Build history of the part. All positions in model axes, mm. A direction names the side the tool comes from. Give positions to 0.01 mm unless a question says otherwise; leave off trailing zeros. Write each loop counter-clockwise with the first axis right and the second up, starting at its lowest first coordinate (ties: lowest second). Pieces come first, ordered by that corner, then holes. Notation, with made-up numbers: M 83,24 L 93,24 A25 cw 93,60 Z; hole C 40.25,64.25 d2. An arc over 180 degrees is marked long. One line per item, written item: value. Start each with the question number.
from build123d import *

# Parameters (mm, degrees)
PAD_DEPTH       = 36.55
SKETCH001_R     = 24.260062
PAD001_DEPTH    = 2
PAD002_DEPTH    = 8
PAD003_START    = 34.55
SKETCH005_R     = 22
SKETCH005_R_2   = 19
PAD003_DEPTH    = 2
SKETCH002_W     = 60
SKETCH002_H     = 10
POCKET002_DEPTH = 36.551
POCKET003_START = 8
SKETCH003_W     = 14
SKETCH003_H     = 60
POCKET003_DEPTH = 52
CHAMFER_SIZE    = 0.99


with BuildPart() as part:
    # Sketch → Pad (new body)
    with BuildSketch(Plane.XY):
        with BuildLine():
            Line((19.47946, 10.225), (22, 10.225))
            Line((22, 10.225), (22, -10.225))
            Line((22, -10.225), (19.47946, -10.225))
            ThreePointArc((10.225, -19.47946), (15.556349, -15.556349), (19.47946, -10.225))
            Line((10.225, -22), (10.225, -19.47946))
            Line((-10.225, -22), (10.225, -22))
            Line((-10.225, -19.47946), (-10.225, -22))
            ThreePointArc((-19.47946, -10.225), (-15.556349, -15.556349), (-10.225, -19.47946))
            Line((-22, -10.225), (-19.47946, -10.225))
            Line((-22, 10.225), (-22, -10.225))
            Line((-19.47946, 10.225), (-22, 10.225))
            ThreePointArc((-10.225, 19.47946), (-15.556349, 15.556349), (-19.47946, 10.225))
            Line((-10.225, 19.47946), (-10.225, 22))
            Line((-10.225, 22), (10.225, 22))
            Line((10.225, 22), (10.225, 19.47946))
            ThreePointArc((19.47946, 10.225), (15.556349, 15.556349), (10.225, 19.47946))
        make_face()
        with BuildLine():
            Line((-20, 0), (-20, 8.225))
            Line((-20, 8.225), (-18.230452, 8.225))
            ThreePointArc((18.230452, 8.225), (0, 20), (-18.230452, 8.225))
            Line((18.230452, 8.225), (20, 8.225))
            Line((20, 8.225), (20, 0.000241))
            Line((20, 0.000241), (20, -8.224518))
            Line((20, -8.224518), (18.230669, -8.224518))
            ThreePointArc((-18.230452, -8.225), (0.000264, -20), (18.230669, -8.224518))
            Line((-20, -8.225), (-18.230452, -8.225))
            Line((-20, 0), (-20, -8.225))
        make_face(mode=Mode.SUBTRACT)
    extrude(amount=PAD_DEPTH)

    # Sketch001 → Pad001 (join)
    with BuildSketch(Plane.XY):
        Circle(SKETCH001_R)
    extrude(amount=-PAD001_DEPTH)

    # Sketch004 → Pad002 (join)
    with BuildSketch(Plane.XY):
        with BuildLine():
            ThreePointArc((-7, 18.734994), (-13.665977, 14.602776), (-18.230452, 8.225))
            Line((-18.230452, 8.225), (-9, 8.225))
            ThreePointArc((-9, 8.225), (-7.585786, 8.810786), (-7, 10.225))
            Line((-7, 10.225), (-7, 18.734994))
        make_face()
        with BuildLine():
            ThreePointArc((18.230452, 8.225), (13.665977, 14.602776), (7, 18.734994))
            Line((7, 18.734994), (7, 10.225))
            ThreePointArc((7, 10.225), (7.585786, 8.810786), (9, 8.225))
            Line((9, 8.225), (18.230452, 8.225))
        make_face()
        with BuildLine():
            ThreePointArc((7, -18.734994), (13.66617, -14.602596), (18.230669, -8.224518))
            Line((18.230669, -8.224518), (9, -8.224518))
            ThreePointArc((9, -8.224518), (7.585786, -8.810305), (7, -10.224518))
            Line((7, -10.224518), (7, -18.734994))
        make_face()
        with BuildLine():
            ThreePointArc((-18.230452, -8.225), (-13.665977, -14.602776), (-7, -18.734994))
            Line((-7, -18.734994), (-7, -10.225))
            ThreePointArc((-7, -10.225), (-7.585786, -8.810786), (-9, -8.225))
            Line((-9, -8.225), (-18.230452, -8.225))
        make_face()
    extrude(amount=PAD002_DEPTH)

    # Sketch005 → Pad003 (join)
    with BuildSketch(Plane.XY.offset(PAD003_START)):
        Circle(SKETCH005_R)
        Circle(SKETCH005_R_2, mode=Mode.SUBTRACT)
    extrude(amount=PAD003_DEPTH)

    # Sketch002 → Pocket002 (cut, through all)
    with BuildSketch(Plane.XY):
        Rectangle(SKETCH002_W, SKETCH002_H)
    extrude(amount=POCKET002_DEPTH, mode=Mode.SUBTRACT)

    # Sketch003 → Pocket003 (cut)
    with BuildSketch(Plane.XY.offset(POCKET003_START)):
        Rectangle(SKETCH003_W, SKETCH003_H)
    extrude(amount=POCKET003_DEPTH, mode=Mode.SUBTRACT)

    # Chamfer
    chamfer_edges = [part.edges().sort_by_distance(p)[0] for p in [
        (-14.159705, 12.668968, 34.55),
        (-14.159705, -12.668968, 34.55),
        (14.159705, 12.668968, 34.55),
        (14.159705, -12.668968, 34.55),
    ]]
    chamfer(chamfer_edges, length=CHAMFER_SIZE)


solid = part.part
1) Probe line 1 along X through (y, z) = (-6.5, 5.5); line 2 along Y through (x, z) = (19.5, 29) (3 decimals); line 3 along X through (y, z) = (-20, 25.5) (3 decimals). List the from-to ranges inside material, lowest first. Write a range as from..to.
2) Tool access for faces 1 (the face through (21, 5, 18)), 2 (the face through (-16, 16, 0)), 3 (the face through (-19, 8.225, 9)), 4 (the face through (-7.57, -8.826, 3.944)): list every direction of +Z, -Z, +X, -X, +Y, -Y with a clear straight run to the whole face (end or side of a thin tool).
3) Mould opens along X. For faces 5 (the face through (22, -8, 18)), 6 (the face through (21, -10.225, 18)), 7 (the face through (7, -14, 4)), 8 (the face through (-22, 8, 18)) say: released by +X, released by -X, zero draft, split by the parting line, or undercut.
4) Band-saw the part on B-B (y = 0). List the corners of the cut face in (x, z), then the cut area to 3 significant figures.
5) Drop flat-ended pins along their axis: P1, Ø1, axis at y = 7, z = 13, coming from the +X side; P2, Ø1.3, axis at y = 20.5, z = 9.5, coming from the -X side (3 decimals); P3, Ø1.3, axis at x = -20, z = 13, coming from the -Y side; P4, Ø13, axis at x = -13, y = 19, coming from the +Z side. Give the stop position or say it passes through.
6) Band-saw the part on A-A (x = 0). List the corners of the cut face in (y, z), then the cut area to 3 significant figures.
Model answer:
1. line 1: x = -22..-20, 20..22
1. line 2: y = -10.225..-8.225, 8.225..10.225
1. line 3: x = -10.225..-7, 7..10.225
2. face 1: +Z, +X, -X
2. face 2: +Z, -X, +Y
2. face 3: none
2. face 4: +Z
3. face 5: released by +X
3. face 6: zero draft
3. face 7: undercut
3. face 8: released by -X
4. outline: M -24.26,-2 L 24.26,-2 L 24.26,0 L -24.26,0 Z
4. area: 97.0 mm²
5. P1: stops at x = 22
5. P2: stops at x = -10.225
5. P3: stops at y = -10.47
5. P4: stops at z = 36.55
6. outline: M -24.26,-2 L 24.26,-2 L 24.26,0 L 22,0 L 22,8 L 20,8 L 20,0 L -20,0 L -20,8 L -22,8 L -22,0 L -24.26,0 Z
6. area: 129 mm²
